Could you check a few things on this drawing? It's one solid part, dimensions in mm from its lowest x, y, z. Give positions to 0.01 mm unless a question says otherwise; leave off trailing zeros. Loops run counter-clockwise (first coordinate to the right, second up) from the corner with the lowest first, then second, coordinate; pieces in that order, holes last. Notation, with made-up numbers: (66, 49.5) - (85, 49.5) arc R32 cw to (85, 76.5) - close; hole circle Ø11 at (86.25, 40). An arc over 180 degrees is marked (long way). Write each question's results on one line, items separated by ' | '. Start each with the question number.
(1) If we mould it in two halves opening along X, with no side actions, what happens to the marked faces 1, 2 and 3? For each: released by +X, released by -X, zero draft, split by the parting line, or undercut.
(2) Suppose I cut it at A-A (x = 10). Please give me the cut outline in (y, z), and give its area (3 significant figures).
(3) Suppose I cut it at D-D (z = 15.25). Please give me the cut outline in (x, y).
(4) Suppose I cut it at B-B (z = 10). Please give me the cut outline in (x, y).
(5) I need wall thicknesses on line 1 (X direction, y = 8.75, z = 10); line 2 (Y direction, x = 1.5, z = 7.25); line 3 (Z direction, x = 10.5, y = 13). Which ranges of each line are inside material? Lowest first, please.
(6) For pin 1 (3 mm diameter, centred on y = 8.5, z = 12, fed in from +X); pin 2 (1.5 mm diameter, centred on x = 6.5, y = 9.5, fed in from -Z); pin 3 (2 mm diameter, centred on x = 16, y = 2.5, fed in from +Z), each with a flat end and sliding along its axis, tell me the tip position at first contact or that it passes through.
(7) Suppose I cut it at C-C (y = 1.5). Please give me the cut outline in (x, z).
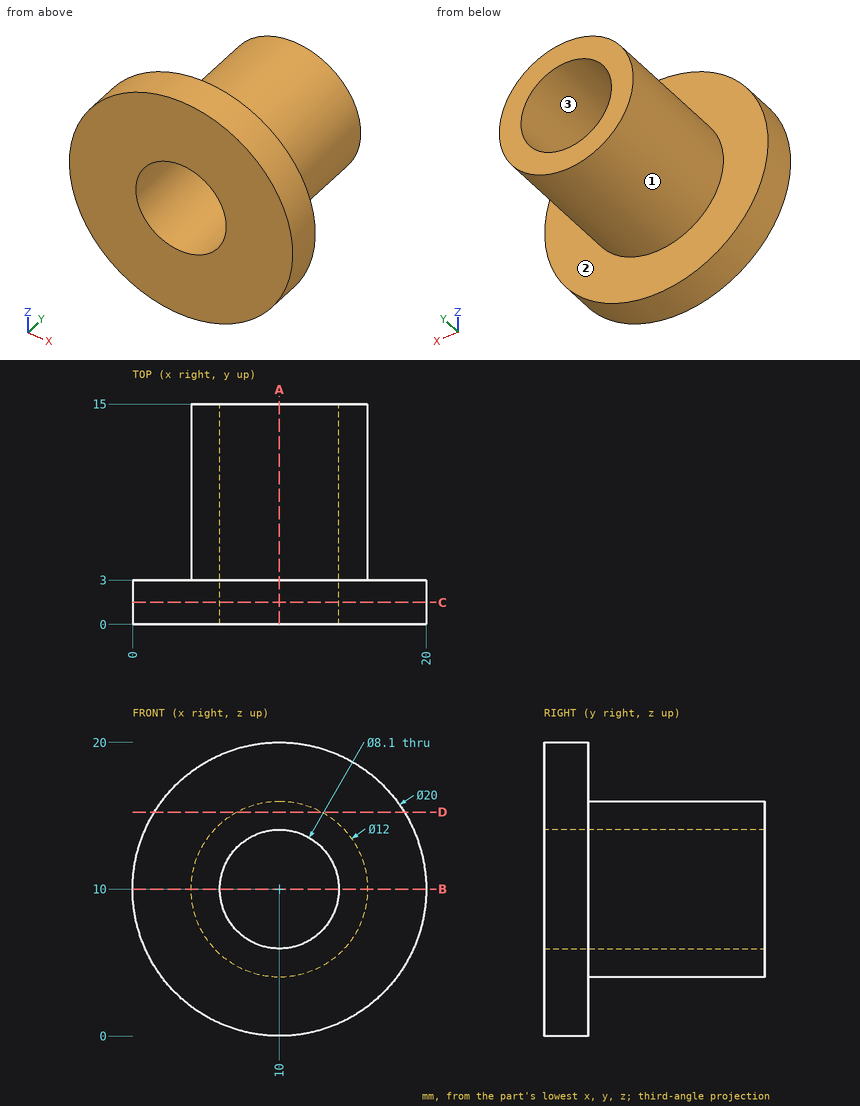
Output values:
1) face 1: split by the parting line | face 2: zero draft | face 3: undercut
2) outline: (0, 0) - (3, 0) - (3, 4) - (15, 4) - (15, 5.95) - (0, 5.95) - close; (0, 14.05) - (15, 14.05) - (15, 16) - (3, 16) - (3, 20) - (0, 20) - close | area: 82.5 mm2
3) outline: (1.49, 0) - (18.51, 0) - (18.51, 3) - (12.9, 3) - (12.9, 15) - (7.1, 15) - (7.1, 3) - (1.49, 3) - close
4) outline: (0, 0) - (5.95, 0) - (5.95, 15) - (4, 15) - (4, 3) - (0, 3) - close; (14.05, 0) - (20, 0) - (20, 3) - (16, 3) - (16, 15) - (14.05, 15) - close
5) line 1: 4 to 5.95, 14.05 to 16 | line 2: 0 to 3 | line 3: 4.02 to 5.98, 14.02 to 15.98
6) pin 1: x = 15.98 | pin 2: z = 4.67 | pin 3: z = 18.66
7) outline: circle Ø20 at (10, 10); hole circle Ø8.1 at (10, 10)
